Check sheet for the drawn part. Datum: minimum x, y, z corner. Units: mm. Round coordinates to 2 decimals unless told otherwise and drop trailing zeros. Write each loop counter-clockwise with the first axis right and the second up, starting at its lowest first coordinate (ties: lowest second). Pieces come first, ordered by that corner, then holes. Notation, with made-up numbers: M 12.25,9 L 66.25,9 A24 ccw 66.25,29 Z; hole C 4,7 d2. An arc over 180 degrees is marked long. Use a Markdown table: item, result.
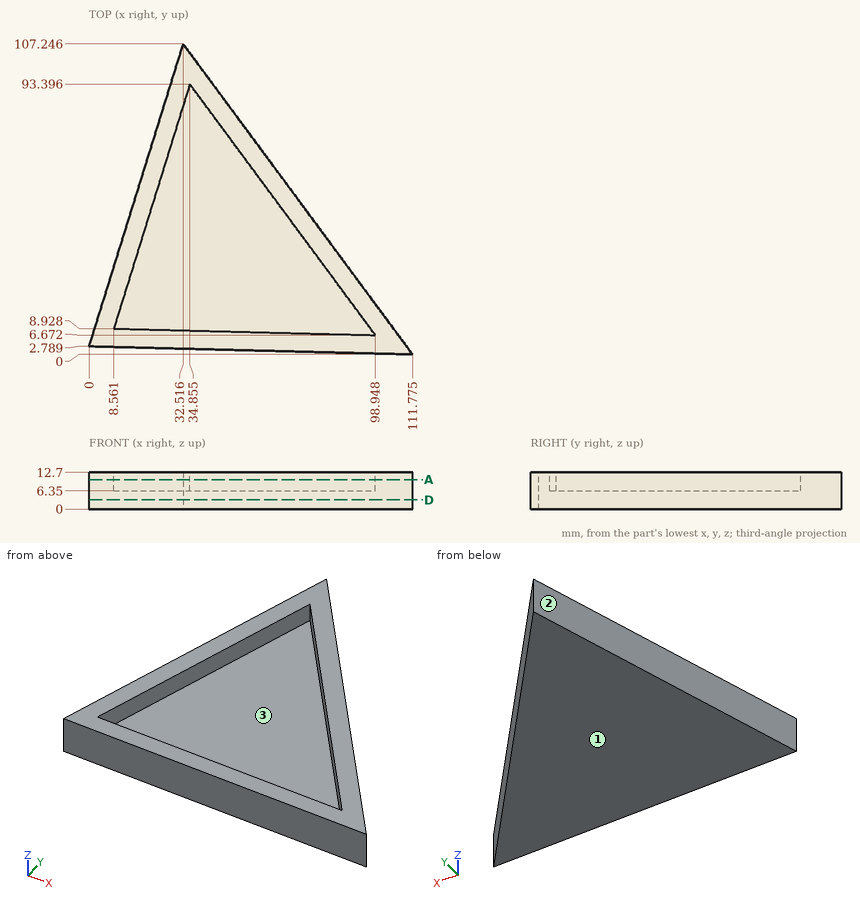
Item 1: Cross-section at A-A, the plane z = 10.25. Record the cut outline in (x, y) (1 decimal), and give its area (3 significant figures).
Outcome:
| item | result |
|---|---|
| outline | M 0,2.8 L 111.8,0 L 32.5,107.2 Z; hole M 8.6,8.9 L 98.9,6.7 L 34.9,93.4 Z |
| area | 2,040 mm2 |
Item 2: Cross-section at D-D, the plane z = 3.25. Record the cut outline in (x, y) (1 decimal).
Outcome:
| item | result |
|---|---|
| outline | M 0,2.8 L 111.8,0 L 32.5,107.2 Z |
Item 3: Material ranges on line 1 along Z through (x, y) = (47, 72.5); line 2 along X through (y, z) = (24.5, 11); line 3 along Y through (x, z) = (73, 7.25) (1 decimal), recorded low to high. Write a range as from..to.
Outcome:
| item | result |
|---|---|
| line 1 | z = 0..6.35 |
| line 2 | x = 6.76..13.41, 85.77..93.67 |
| line 3 | y = 1..7.3, 41.8..52.5 |
Item 4: Mould release check, pull along X, two halves, no side actions. Record for the marked faces 1, 2 and 3: +X half, -X half, draft (parallel to the pull), parting line (faces both ways), or undercut.
Outcome:
| item | result |
|---|---|
| face 1 | draft |
| face 2 | -X half |
| face 3 | undercut |
Item 5: Go/stop test with flat-tipped pins: pin 1 (4 mm diameter, centred on y = 49, z = 4.5, fed in from -X); pin 2 (1.5 mm diameter, centred on y = 89, z = 7.5, fed in from -X); pin 3 (5 mm diameter, centred on y = 23.5, z = 3.5, fed in from -X). Record where each tip stops, or that it passes through.
Outcome:
| item | result |
|---|---|
| pin 1 | stops at x = 13.76 |
| pin 2 | stops at x = 26.6 |
| pin 3 | stops at x = 5.67 |
